```python
from build123d import *

# Parameters (mm, degrees)
SKETCH_1_R      = 2.1
EXTRUDE_1_DEPTH = 3
SKETCH_2_R      = 3
SKETCH_2_R_2    = 2.1
EXTRUDE_2_DEPTH = 0.2


with BuildPart() as part:
    # 草图1 → 凸台-拉伸1 (new body)
    with BuildSketch(Plane.XY):
        with BuildLine():
            Line((0, 7.5), (14, 7.5))
            ThreePointArc((14, 7.5), (21.5, 0), (14, -7.5))
            Line((14, -7.5), (0, -7.5))
            ThreePointArc((0, -7.5), (-7.5, 0), (0, 7.5))
        make_face()
        Circle(SKETCH_1_R, mode=Mode.SUBTRACT)
        with Locations((14, 0)):
            Circle(SKETCH_1_R, mode=Mode.SUBTRACT)
    extrude(amount=EXTRUDE_1_DEPTH)

    # 草图2 → 凸台-拉伸2 (add)
    # profile 1 of 2: a face of its own
    with BuildSketch(Plane.XY.offset(3)):
        Circle(SKETCH_2_R)
        Circle(SKETCH_2_R_2, mode=Mode.SUBTRACT)
    # profile 2 of 2: a face of its own
    with BuildSketch(Plane.XY.offset(3)):
        with Locations((14, 0)):
            Circle(SKETCH_2_R)
        with Locations((14, 0)):
            Circle(SKETCH_2_R_2, mode=Mode.SUBTRACT)
    extrude(amount=EXTRUDE_2_DEPTH)


solid = part.part
```
Input: part model. Units: mm. Frame: model coordinates. A direction names the side the tool comes from. Give positions to 0.01 mm unless a question says otherwise; leave off trailing zeros. Loops run counter-clockwise (first coordinate to the right, second up) from the corner with the lowest first, then second, coordinate; pieces in that order, holes last. Notation, with made-up numbers: (-8.5, -26) -> (14.5, -26) arc R21 cw to (14.5, -2) -> close; hole circle Ø1 at (83.5, 9). An arc over 180 degrees is marked (long way). Use a Markdown table: item, result.
Q1. First-contact query: P1, Ø1.5, axis at x = -4.5, y = -4, coming from the +Z side; P2, Ø1.5, axis at x = 15, z = 1, coming from the -Y side. Flat tips, straight axial feed; report the tip coordinate or a pass-through.
Entries:
| item | result |
|---|---|
| P1 | stops at z = 3 |
| P2 | stops at y = -7.5 |
Q2. Section query D-D, the plane x = 9. Return the cut outline in (y, z), plus the area to 3 significant figures.
Entries:
| item | result |
|---|---|
| outline | (-7.5, 0) -> (7.5, 0) -> (7.5, 3) -> (-7.5, 3) -> close |
| area | 45.0 mm² |
Q3. Ray query, probe 1 along X at (y, z) = (1.5, 1.55); probe 2 along Y at (x, z) = (0, 1.25); probe 3 along X at (y, z) = (-1.25, 1.7). Return the intervals inside material, ascending. Write a range as from..to.
Entries:
| item | result |
|---|---|
| probe 1 | x = -7.35..-1.47, 1.47..12.53, 15.47..21.35 |
| probe 2 | y = -7.5..-2.1, 2.1..7.5 |
| probe 3 | x = -7.4..-1.69, 1.69..12.31, 15.69..21.4 |
Q4. Pull-direction query (X, two-part tool) for faces 3 (the cylindrical face through (2.003, 0.631, 1.578)), 4 (the cylindrical face through (-7.5, -0.16, 1.48)), 5 (the flat face through (1.3, -2, 3.2)); classes: pulls with the +X half, pulls with the -X half, needs draft (parallel to the pull), parting line crosses it, or undercut.
Entries:
| item | result |
|---|---|
| face 3 | undercut |
| face 4 | pulls with the -X half |
| face 5 | needs draft |
Q5. Section query C-C, the plane z = 2.15. Return the cut outline in (x, y).
Entries:
| item | result |
|---|---|
| outline | (0, -7.5) -> (14, -7.5) arc R7.5 ccw to (14, 7.5) -> (0, 7.5) arc R7.5 ccw to start; hole circle Ø4.2 at (0, 0); hole circle Ø4.2 at (14, 0) |
Q6. Section query A-A, the plane y = 0. Return the cut outline in (x, z).
Entries:
| item | result |
|---|---|
| outline | (-7.5, 0) -> (-2.1, 0) -> (-2.1, 3.2) -> (-3, 3.2) -> (-3, 3) -> (-7.5, 3) -> close; (2.1, 0) -> (11.9, 0) -> (11.9, 3.2) -> (11, 3.2) -> (11, 3) -> (3, 3) -> (3, 3.2) -> (2.1, 3.2) -> close; (16.1, 0) -> (21.5, 0) -> (21.5, 3) -> (17, 3) -> (17, 3.2) -> (16.1, 3.2) -> close |
Q7. Section query B-B, the plane x = 0.75. Return the cut outline in (y, z).
Entries:
| item | result |
|---|---|
| outline | (-7.5, 0) -> (-1.96, 0) -> (-1.96, 3.2) -> (-2.9, 3.2) -> (-2.9, 3) -> (-7.5, 3) -> close; (1.96, 0) -> (7.5, 0) -> (7.5, 3) -> (2.9, 3) -> (2.9, 3.2) -> (1.96, 3.2) -> close |
Q8. Access query for faces 1 (the flat face through (7, 7.5, 1)), 2 (the flat face through (7, 0, 3)). Directions: +Z, -Z, +X, -X, +Y, -Y. A direction counts if a zero-diameter tool reaches every point of the face in a straight line with its end or side. Return the directions, or none.
Entries:
| item | result |
|---|---|
| face 1 | +Z, -Z, +X, -X, +Y |
| face 2 | +Z |
